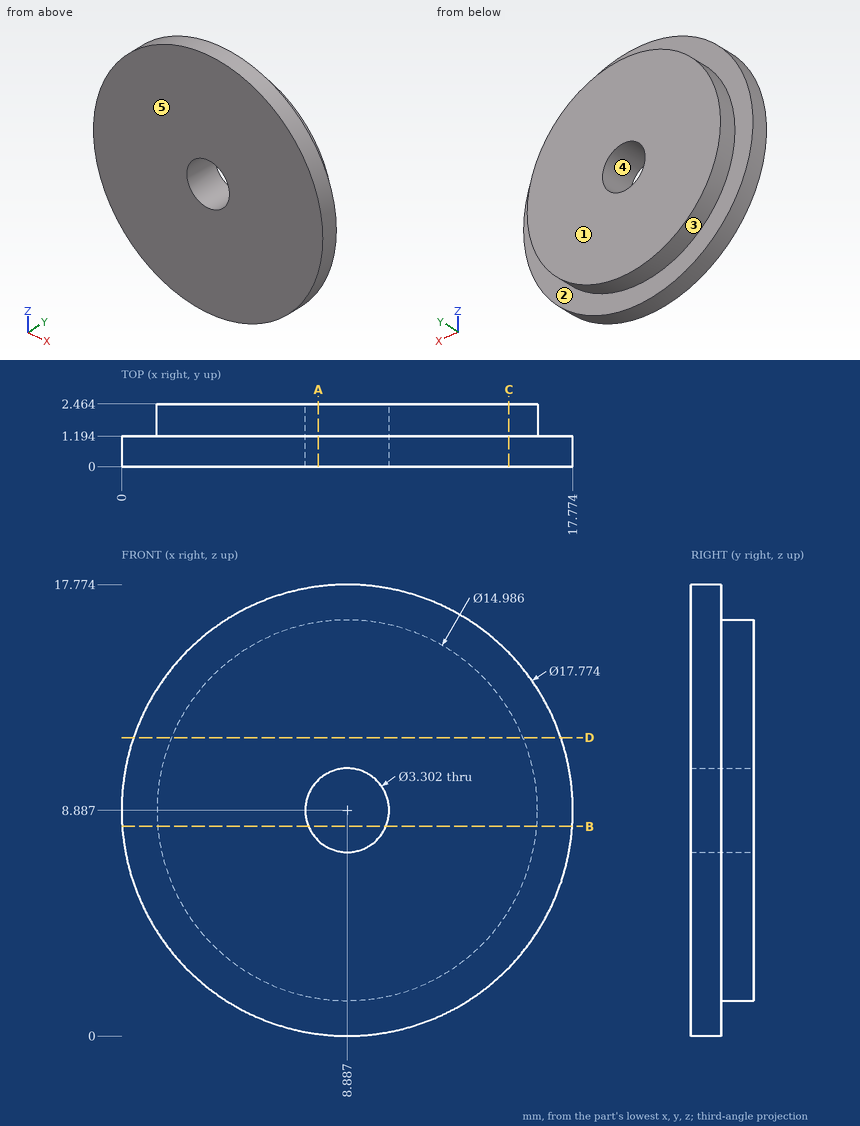
Part print with two shaded views. Sizes in mm from the minimum x, y, z corner. A direction names the side the tool comes from. Round coordinates to 2 decimals unless told otherwise and drop trailing zeros. Loops run counter-clockwise (first coordinate to the right, second up) from the corner with the lowest first, then second, coordinate; pieces in that order, holes last.
Item 1: Saw through at C-C (x = 15.25). List the corners of the cut face in (y, z), then the cut area to 3 significant figures.
Item 2: Saw through at D-D (z = 11.75). List the corners of the cut face in (x, y).
Item 3: Saw through at B-B (z = 8.25). List the corners of the cut face in (x, y).
Item 4: Drill centre lines: line 1 along Y through (x, z) = (8.75, 1); line 2 along X through (y, z) = (1.25, 7.75) (1 decimal); line 3 along Z through (x, y) = (3.5, 1.4) (1 decimal). Where is each one in solid material? Low to high.
Item 5: Saw through at A-A (x = 7.75). List the corners of the cut face in (y, z).
Item 6: Two-plate mould, pull along Z, no slides. Class the marked faces 3, 4 and 5: released by +Z, released by -Z, zero draft, split by the parting line, or undercut.
Item 7: Which spindle directions (+Z, -Z, +X, -X, +Y, -Y) get a long thin tool onto all of the face, cutting with end or side? Do the marked faces 1 and 2. Say none if no direction does.
Worked answers:
1. outline: (0, 2.68) - (1.19, 2.68) - (1.19, 4.93) - (2.46, 4.93) - (2.46, 12.84) - (1.19, 12.84) - (1.19, 15.09) - (0, 15.09) - close
1. area: 24.9 mm2
2. outline: (0.47, 0) - (17.3, 0) - (17.3, 1.19) - (15.81, 1.19) - (15.81, 2.46) - (1.96, 2.46) - (1.96, 1.19) - (0.47, 1.19) - close
3. outline: (0.02, 0) - (7.36, 0) - (7.36, 2.46) - (1.42, 2.46) - (1.42, 1.19) - (0.02, 1.19) - close; (10.41, 0) - (17.75, 0) - (17.75, 1.19) - (16.35, 1.19) - (16.35, 2.46) - (10.41, 2.46) - close
4. line 1: y = 0 to 1.19
4. line 2: x = 1.5 to 7.7, 10.1 to 16.3
4. line 3: z = 3.7 to 14.1
5. outline: (0, 0.07) - (1.19, 0.07) - (1.19, 1.48) - (2.46, 1.48) - (2.46, 7.69) - (0, 7.69) - close; (0, 10.08) - (2.46, 10.08) - (2.46, 16.29) - (1.19, 16.29) - (1.19, 17.7) - (0, 17.7) - close
6. face 3: split by the parting line
6. face 4: undercut
6. face 5: zero draft
7. face 1: +Z, -Z, +X, -X, +Y
7. face 2: +Y
